The figure shows three views and two pictorial views of one solid part (mm, origin at its lowest corner). Answer the questions. A direction names the side the tool comes from. Coordinates: 2 decimals unless noted, no trailing zeros. Write each loop counter-clockwise with the first axis right and the second up, starting at its lowest first coordinate (ties: lowest second). Pieces come first, ordered by that corner, then holes. Notation, with made-up numbers: (-39.5, 9.25) - (-16.5, 9.25) arc R19 ccw to (-16.5, 36.25) - close; hole circle Ø2 at (-30, -25). An arc over 180 degrees is marked (long way). Use a Markdown table: item, result. Add a question column.
(1) For a pull along X with two mould halves and no side action, classify the marked faces 5, 6, 7 and 8 as released by +X, released by -X, zero draft, split by the parting line, or undercut.
(2) The part is cut by section A-A, the plane y = 5. Give the vertices of the cut face in (x, z).
(3) Given pin 1 Ø8 at (y, z) = (6, 8) entering from +X; pin 2 Ø6 at (x, y) = (21, 8) entering from +Z; pin 3 Ø6.5 at (x, z) = (6, 11.5) entering from +Y, each flat-ended and moving along its own axis, determine where each tip first touches the part or whether it passes through.
(4) A tool of negligible diameter and unlimited length cuts with its end or side. For the marked faces 1, 2, 3 and 4, from which of +Z, -Z, +X, -X, +Y, -Y can it reach the whole face along a straight path? Write none if from no direction.
(5) Find the intervals of material crossed by line 1 (X direction, y = 1.75, z = 11.25); line 2 (Y direction, x = 35, z = 3.25); line 3 (Z direction, x = 5.5, y = 3.5), in increasing order. Write a range as from..to.
(6) The part is cut by section C-C, the plane z = 15.25. Give the vertices of the cut face in (x, y).
(7) The part is cut by section B-B, the plane x = 38. Give the vertices of the cut face in (y, z), then the cut area to 3 significant figures.
(8) The part is cut by section D-D, the plane z = 8.5. Give the vertices of the cut face in (x, y), then the cut area to 3 significant figures.
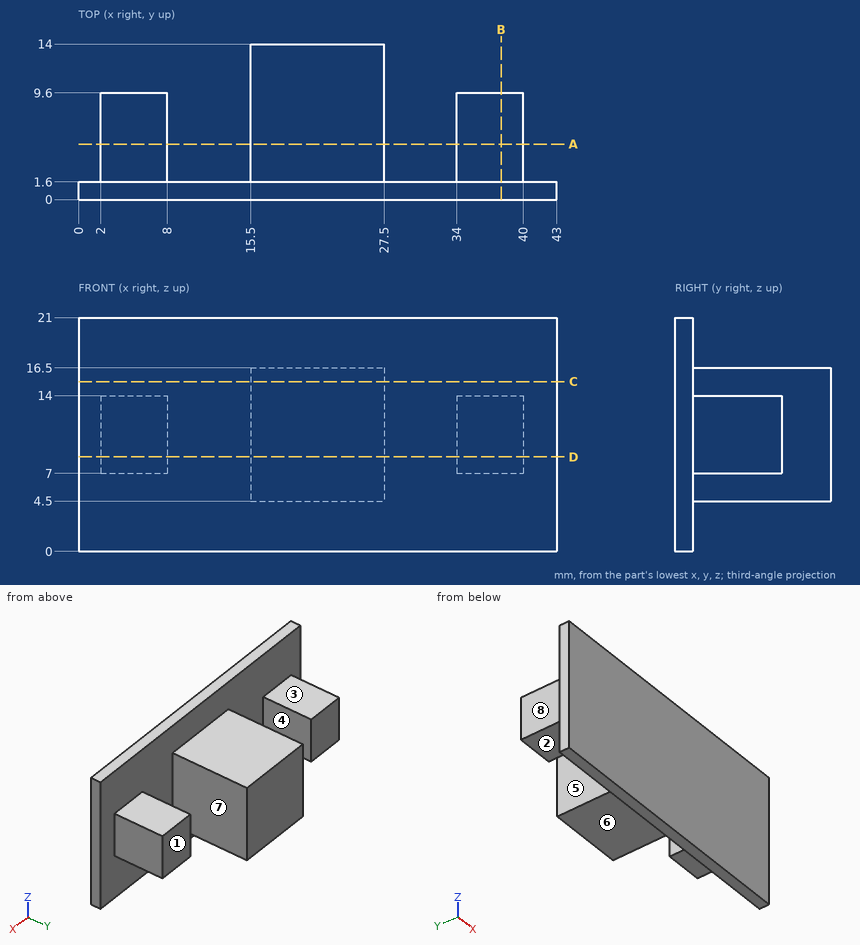
Model answer:
| question | item | result |
|---|---|---|
| 1 | face 5 | undercut |
| 1 | face 6 | zero draft |
| 1 | face 7 | undercut |
| 1 | face 8 | released by -X |
| 2 | outline | (2, 7) - (8, 7) - (8, 14) - (2, 14) - close; (15.5, 4.5) - (27.5, 4.5) - (27.5, 16.5) - (15.5, 16.5) - close; (34, 7) - (40, 7) - (40, 14) - (34, 14) - close |
| 3 | pin 1 | x = 40 |
| 3 | pin 2 | z = 16.5 |
| 3 | pin 3 | y = 9.6 |
| 4 | face 1 | +Z, -Z, +X, +Y |
| 4 | face 2 | -Z, -X, +Y |
| 4 | face 3 | +Z, -X, +Y |
| 4 | face 4 | +Z, -Z, +Y |
| 5 | line 1 | 2..8, 15.5..27.5, 34..40 |
| 5 | line 2 | 0..1.6 |
| 5 | line 3 | 7..14 |
| 6 | outline | (0, 0) - (43, 0) - (43, 1.6) - (27.5, 1.6) - (27.5, 14) - (15.5, 14) - (15.5, 1.6) - (0, 1.6) - close |
| 7 | outline | (0, 0) - (1.6, 0) - (1.6, 7) - (9.6, 7) - (9.6, 14) - (1.6, 14) - (1.6, 21) - (0, 21) - close |
| 7 | area | 89.6 mm^2 |
| 8 | outline | (0, 0) - (43, 0) - (43, 1.6) - (40, 1.6) - (40, 9.6) - (34, 9.6) - (34, 1.6) - (27.5, 1.6) - (27.5, 14) - (15.5, 14) - (15.5, 1.6) - (8, 1.6) - (8, 9.6) - (2, 9.6) - (2, 1.6) - (0, 1.6) - close |
| 8 | area | 314 mm^2 |
